The listing builds one solid part. Answer for the finished solid, in the listing's coordinates (mm). Face numbers are marked on the shaded views. A direction names the side the tool comes from. Give positions to 0.01 mm unless a question says otherwise; leave off trailing zeros. Order: outer loops, then holes, each group sorted by start corner. A loop starts at its lowest first (then second) coordinate and runs counter-clockwise, first axis right, second up. Notation, with made-up numbers: (75.25, 82) - (116.25, 82) arc R31 cw to (116.25, 107) - close; hole circle Ø9 at (57, 85.25). An arc over 180 degrees is marked (long way). Answer in a Markdown table with one row per item.
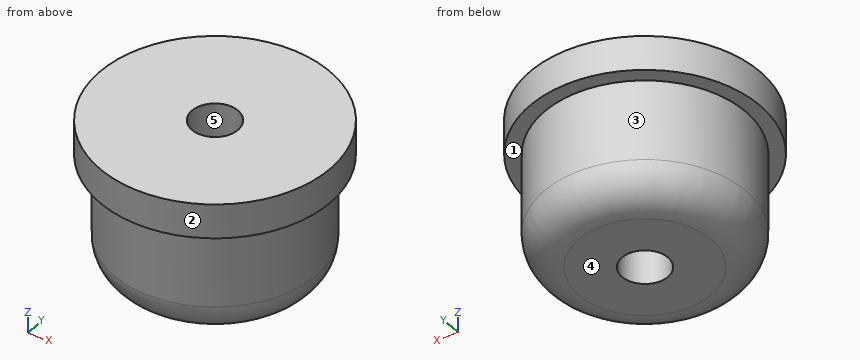
from build123d import *

# Parameters (mm, degrees)
F0_R     = 10
F1_DEPTH = 3
F2_R     = 8.75
F3_DEPTH = 10
F4_R     = 3
F6_D     = 4


with BuildPart() as f1:
    # F0 (on Top) → F1 (new body)
    with BuildSketch(Plane.XY):
        Circle(F0_R)
    extrude(amount=F1_DEPTH)

    # F2 (on face) → F3 (join)
    with BuildSketch(Plane(origin=(0, 0, 0), x_dir=(1, 0, 0), z_dir=(0, 0, -1))):
        Circle(F2_R)
    extrude(amount=F3_DEPTH)

    # F4
    f4_edges = [f1.edges().sort_by_distance(p)[0] for p in [
        (-8.75, 0, -10),
    ]]
    fillet(f4_edges, radius=F4_R)

    # F6 (through all)
    with Locations(Plane(origin=(0, 0, -10), x_dir=(1, 0, 0), z_dir=(0, 0, -1))):
        with Locations((0, 0)):
            Hole(F6_D / 2)


solid = f1.part
Item 1: Which of the six approach directions +Z, -Z, +X, -X, +Y, -Y give full straight-line access (tool end or side, diameter ignored) to the marked faces 1 and 2?
Answer block:
| item | result |
|---|---|
| face 1 | -Z |
| face 2 | +Z, -Z |
Item 2: Find section D-D on z = -2.75. Write down the section's boundary in (x, y).
Answer block:
| item | result |
|---|---|
| outline | circle Ø17.5 at (0, 0); hole circle Ø4 at (0, 0) |
Item 3: Consider line 1 (Y direction, x = 0, z = -7); line 2 (X direction, y = -1.25, z = -4); line 3 (X direction, y = 1, z = 1.25). Determine where each line is inside the solid, lowest interval first.
Answer block:
| item | result |
|---|---|
| line 1 | -8.75 to -2, 2 to 8.75 |
| line 2 | -8.66 to -1.56, 1.56 to 8.66 |
| line 3 | -9.95 to -1.73, 1.73 to 9.95 |
Item 4: Determine the mould class of the marked faces 3, 4 and 5 for opening direction X: pulls with the +X half, pulls with the -X half, needs draft (parallel to the pull), parting line crosses it, or undercut.
Answer block:
| item | result |
|---|---|
| face 3 | parting line crosses it |
| face 4 | needs draft |
| face 5 | undercut |
Item 5: Each of these flat-tipped pins is pushed along its axis until it touches: P1, Ø5, axis at y = -2, z = -5.5, coming from the +X side; P2, Ø5, axis at y = -1.5, z = -4.5, coming from the -X side; P3, Ø2, axis at x = 2, z = -7, coming from the -Y side. Where does it stop, or does it pass through?
Answer block:
| item | result |
|---|---|
| P1 | x = 8.75 |
| P2 | x = -8.75 |
| P3 | y = -8.69 |
Item 6: Find section C-C on z = 1.5. Write down the section's boundary in (x, y), then the cut area to 3 significant figures.
Answer block:
| item | result |
|---|---|
| outline | circle Ø20 at (0, 0); hole circle Ø4 at (0, 0) |
| area | 302 mm² |
Item 7: Find section A-A on x = 0. Write down the section's boundary in (y, z), then the cut area to 3 significant figures.
Answer block:
| item | result |
|---|---|
| outline | (-10, 0) - (-8.75, 0) - (-8.75, -7) arc R3 ccw to (-5.75, -10) - (-2, -10) - (-2, 3) - (-10, 3) - close; (2, -10) - (5.75, -10) arc R3 ccw to (8.75, -7) - (8.75, 0) - (10, 0) - (10, 3) - (2, 3) - close |
| area | 179 mm² |
